Study the drawing (mm; zero at the part's minimum x, y, z) and answer. A direction names the side the tool comes from. Round coordinates to 2 decimals unless told otherwise and drop trailing zeros. Loops run counter-clockwise (first coordinate to the right, second up) from the corner with the lowest first, then second, coordinate; pieces in that order, holes last. Notation, with made-up numbers: (88.25, -7.75) - (142.25, -7.75) arc R21 cw to (142.25, 4.25) - close; hole circle Ø1 at (2.5, -6.5). An arc over 180 degrees is marked (long way). One line per item, written item: value.
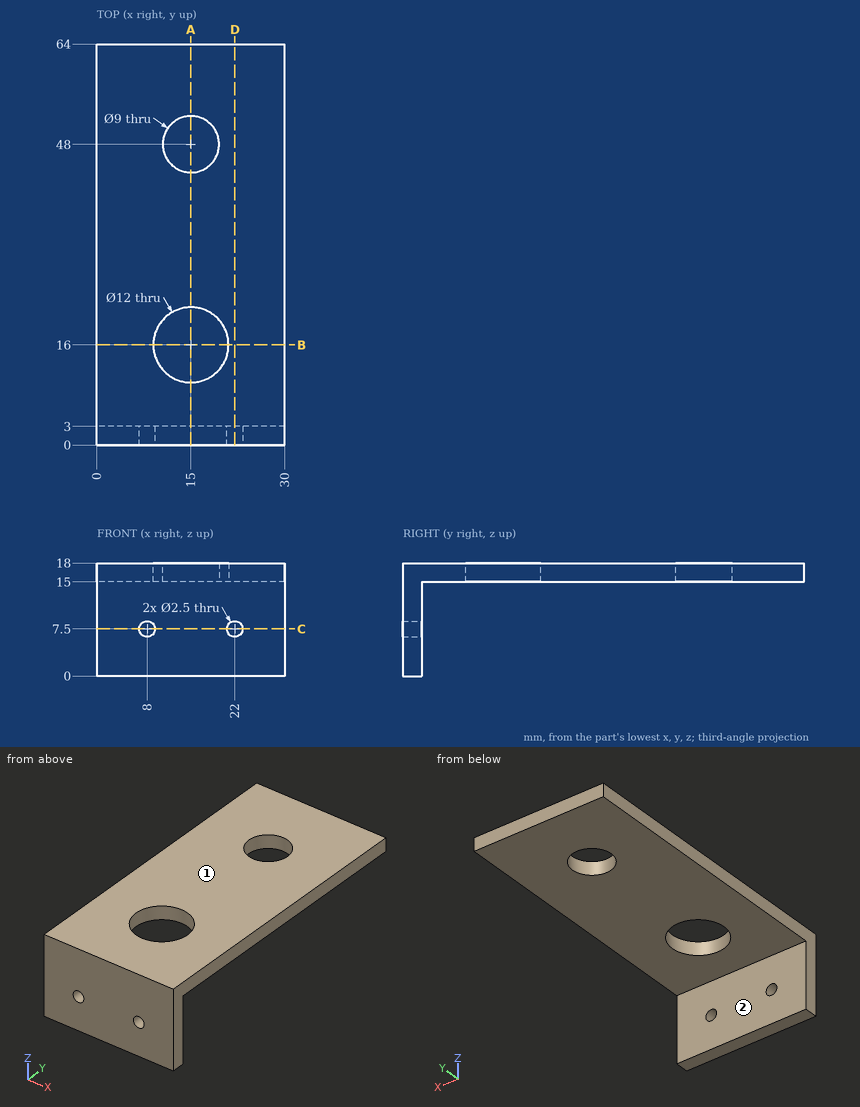
1) A cutting plane is placed at B-B on y = 16. Give the vertices of the cut face in (x, z).
Final values:
outline: (0, 15) - (9, 15) - (9, 18) - (0, 18) - close; (21, 15) - (30, 15) - (30, 18) - (21, 18) - close
2) Each of these flat-tipped pins is pushed along its axis until it touches: pin 1 Ø8 at (x, y) = (22, 42.5) entering from -Z; pin 2 Ø1.5 at (x, z) = (22, 7.5) entering from -Y; pin 3 Ø3 at (x, z) = (8, 7.5) entering from -Y; pin 4 Ø4.5 at (x, z) = (9, 6.5) entering from +Y. Where does it stop, or does it pass through?
Final values:
pin 1: z = 15
pin 2: through
pin 3: y = 0
pin 4: y = 3
3) A cutting plane is placed at C-C on z = 7.5. Give the vertices of the cut face in (x, y).
Final values:
outline: (0, 0) - (6.75, 0) - (6.75, 3) - (0, 3) - close; (9.25, 0) - (20.75, 0) - (20.75, 3) - (9.25, 3) - close; (23.25, 0) - (30, 0) - (30, 3) - (23.25, 3) - close
4) For the marked faces 1 and 2, determine the directions among +Z, -Z, +X, -X, +Y, -Y from which every point of the face is accessible in a straight line to the end or side of a thin tool.
Final values:
face 1: +Z, +X, -X, +Y, -Y
face 2: -Z, +X, -X, +Y
5) A cutting plane is placed at D-D on x = 22. Give the vertices of the cut face in (y, z), and give its area (4 significant figures).
Final values:
outline: (0, 0) - (3, 0) - (3, 6.25) - (0, 6.25) - close; (0, 8.75) - (3, 8.75) - (3, 15) - (64, 15) - (64, 18) - (0, 18) - close
area: 229.5 mm2
6) Consider L1, parallel to Y at x = 15, z = 15.7; L2, parallel to X at y = 1.25, z = 7.5; L3, parallel to Z at x = 8, y = 2. Determine where each line is inside the solid, lowest interval first.
Final values:
L1: 0 to 10, 22 to 43.5, 52.5 to 64
L2: 0 to 6.75, 9.25 to 20.75, 23.25 to 30
L3: 0 to 6.25, 8.75 to 18
7) A cutting plane is placed at A-A on x = 15. Give the vertices of the cut face in (y, z), and give its area (3 significant figures).
Final values:
outline: (0, 0) - (3, 0) - (3, 15) - (10, 15) - (10, 18) - (0, 18) - close; (22, 15) - (43.5, 15) - (43.5, 18) - (22, 18) - close; (52.5, 15) - (64, 15) - (64, 18) - (52.5, 18) - close
area: 174 mm2
